Model file for the job. Use its own axes, mm. A direction names the side the tool comes from. Give positions to 0.01 mm unless a question says otherwise; leave off trailing zeros. Loops run counter-clockwise (first coordinate to the right, second up) from the corner with the lowest first, then second, coordinate; pieces in that order, holes last. Notation, with made-up numbers: (31, -39.5) -> (42, -39.5) arc R26 ccw to (42, -21.5) -> close; hole circle Ø6 at (27, 20). An arc over 180 degrees is marked (long way). Use CSV: the item, a comma, the result in double quotes. Start each with the question number.
(1) Cut at A-A on x = -38. Write the cut outline in (y, z), then the cut area to 3 significant figures.
(2) Cut at D-D on z = 58.42. Write the cut outline in (x, y) (3 decimals).
(3) Flat gauge pins, fed straight in: pin 1 (1.4 mm diameter, centred on x = -2, z = 53, fed in from -Y); pin 2 (1 mm diameter, centred on x = -2, y = 1, fed in from +Z); pin 3 (11 mm diameter, centred on y = -20, z = 14, fed in from -X); pin 4 (1 mm diameter, centred on y = -28, z = 19.5, fed in from +X). Where does each tip first touch, or does it go through?
(4) Drill centre lines: probe 1 along X at (y, z) = (-31.5, 11.5); probe 2 along Y at (x, z) = (-26.5, 37.5); probe 3 along Z at (x, y) = (-43, -7.5). Where is each one in solid material? Low to high.
(5) 3-axis set-ups, long thin cutter, end or side, ignore diameter. For faces 1 (the flat face through (-2, -19, 43.18)), 2 (the cylindrical face through (5.924, -16.217, 13.555)), 3 (the cylindrical face through (-51.48, -13.872, 16.349)): which of +Z, -Z, +X, -X, +Y, -Y reach the whole face in a straight line?
(6) Pull direction X, two halves, no side cores. Call faces 4 (the flat face through (-22, 0, 38)), 5 (the conical face through (-43.119, 1.265, 76.464)), 6 (the flat face through (0, -22, 21.3)): pulls with the +X half, pulls with the -X half, needs draft (parallel to the pull), parting line crosses it, or undercut.
(7) Cut at B-B on z = 17.78. Write the cut outline in (x, y), then the cut area to 3 significant figures.
(8) Cut at C-C on y = -12. Write the cut outline in (x, z).
from build123d import *

# Parameters (mm, degrees)
BOSS_EXTRUDE1_DEPTH = 77.47
SKETCH2_W           = 43.18
SKETCH2_H           = 44.45
BOSS_EXTRUDE2_DEPTH = 3.81
SKETCH3_R           = 3.81
SKETCH3_R_2         = 1.27
CUT_EXTRUDE1_DEPTH  = 3.81
SKETCH4_R           = 4.7625
BOSS_EXTRUDE3_DEPTH = 12.7
BOSS_EXTRUDE4_START = 12.7
SKETCH5_R           = 4.7625
BOSS_EXTRUDE4_DEPTH = 12.7
FILLET1_R           = 1.016
SKETCH6_W           = 1.27
SKETCH6_H           = 38.1
CUT_EXTRUDE2_DEPTH  = 1.27
FILLET2_R           = 5.08
CHAMFER1_SIZE       = 2.54


with BuildPart() as part:
    # Sketch1 → Boss-Extrude1 (new body)
    with BuildSketch(Plane.XY):
        Polygon((0, 0), (-41.91, 0), (-41.91, -36.83), (0, -36.83), (0, -40.64), (-41.91, -40.64), (-45.72, -40.64), (-45.72, 0), (-45.72, 3.81), (0, 3.81), align=None)
    extrude(amount=BOSS_EXTRUDE1_DEPTH)

    # Sketch2 → Boss-Extrude2 (add)
    with BuildSketch(Plane(origin=(0, 0, 0), x_dir=(0, 0, -1), z_dir=(1, 0, 0))):
        with Locations((-21.59, -18.415)):
            Rectangle(SKETCH2_W, SKETCH2_H)
    extrude(amount=-BOSS_EXTRUDE2_DEPTH)

    # Sketch3 → Cut-Extrude1 (cut)
    with BuildSketch(Plane.ZY.offset(45.72)):
        with Locations(Location((58.42, -18.415, 0), (0, 0, 270))):
            Circle(SKETCH3_R)
        with Locations(Location((47.244, -7.239, 0), (0, 0, 270))):
            Circle(SKETCH3_R_2)
        with Locations(Location((69.596, -7.239, 0), (0, 0, 270))):
            Circle(SKETCH3_R_2)
        with Locations(Location((69.596, -29.591, 0), (0, 0, 270))):
            Circle(SKETCH3_R_2)
        with Locations(Location((47.244, -29.591, 0), (0, 0, 270))):
            Circle(SKETCH3_R_2)
    extrude(amount=-CUT_EXTRUDE1_DEPTH, mode=Mode.SUBTRACT)

    # Sketch4 → Boss-Extrude3 (add)
    with BuildSketch(Plane.ZY.offset(45.72)):
        with Locations(Location((17.78, -18.415, 0), (0, 0, 90))):
            Circle(SKETCH4_R)
    extrude(amount=BOSS_EXTRUDE3_DEPTH)

    # Sketch5 → Boss-Extrude4 (add)
    with BuildSketch(Plane(origin=(0, 0, 0), x_dir=(0, 0, -1), z_dir=(1, 0, 0)).offset(BOSS_EXTRUDE4_START)):
        with Locations(Location((-17.78, -18.415, 0), (0, 0, 90))):
            Circle(SKETCH5_R)
    extrude(amount=-BOSS_EXTRUDE4_DEPTH)

    # Fillet1
    fillet1_edges = [part.edges().sort_by_distance(p)[0] for p in [
        (-58.42, -23.1775, 17.78),
        (12.7, -23.1775, 17.78),
    ]]
    fillet(fillet1_edges, radius=FILLET1_R)

    # Sketch6 → Cut-Extrude2 (cut)
    with BuildSketch(Plane.XZ):
        with Locations((-1.905, 58.42)):
            Rectangle(SKETCH6_W, SKETCH6_H)
    cut_extrude2 = extrude(amount=-CUT_EXTRUDE2_DEPTH, mode=Mode.SUBTRACT)

    # Mirror1: Cut-Extrude2 across plane
    add(cut_extrude2.mirror(Plane(origin=(0, -18.415, 0), x_dir=(0, 0, 1), z_dir=(0, -1, 0))), mode=Mode.SUBTRACT)

    # Fillet2
    fillet2_edges = [part.edges().sort_by_distance(p)[0] for p in [
        (-45.72, 3.81, 38.735),
        (0, 3.81, 38.735),
        (0, -40.64, 38.735),
        (-45.72, -40.64, 38.735),
    ]]
    fillet(fillet2_edges, radius=FILLET2_R)

    # Chamfer1
    chamfer1_edges = [part.edges().sort_by_distance(p)[0] for p in [
        (-1.969148027, -39.576092628, 77.47),
        (-22.86, -40.64, 77.47),
        (-44.232102448, -39.152102448, 77.47),
        (-45.72, -18.415, 77.47),
        (-1.969148027, 2.746092628, 77.47),
        (-44.232102448, 2.322102448, 77.47),
        (-22.86, 3.81, 77.47),
    ]]
    chamfer(chamfer1_edges, length=CHAMFER1_SIZE)


solid = part.part
Check result:
1,outline,"(-40.64, 0) -> (-36.83, 0) -> (-36.83, 77.47) -> (-38.1, 77.47) -> (-40.64, 74.93) -> close; (0, 0) -> (3.81, 0) -> (3.81, 74.93) -> (1.27, 77.47) -> (0, 77.47) -> close"
1,area,"584 mm²"
2,outline,"(-45.72, -35.56) arc R5.08 ccw to (-40.64, -40.64) -> (-5.08, -40.64) arc R5.08 ccw to (-0.161, -36.83) -> (-1.27, -36.83) -> (-1.27, -38.1) -> (-2.54, -38.1) -> (-2.54, -36.83) -> (-41.91, -36.83) -> (-41.91, -22.225) -> (-45.72, -22.225) -> close; (-45.72, -14.605) -> (-41.91, -14.605) -> (-41.91, 0) -> (-2.54, 0) -> (-2.54, 1.27) -> (-1.27, 1.27) -> (-1.27, 0) -> (-0.161, 0) arc R5.08 ccw to (-5.08, 3.81) -> (-40.64, 3.81) arc R5.08 ccw to (-45.72, -1.27) -> close"
3,pin 1,"y = -40.05"
3,pin 2,"z = 76.33"
3,pin 3,"x = -58.42"
3,pin 4,"x = 0"
4,probe 1,"-45.72 to -41.91, -3.81 to 0"
4,probe 2,"-40.64 to -36.83, 0 to 3.81"
4,probe 3,"0 to 46, 48.49 to 68.35, 70.84 to 77.47"
5,face 1,"+Z, +X"
5,face 2,"+X"
5,face 3,"-X"
6,face 4,"undercut"
6,face 5,"pulls with the -X half"
6,face 6,"pulls with the +X half"
7,outline,"(-58.42, -22.16) arc R1.02 ccw to (-57.4, -23.18) -> (-45.72, -23.18) -> (-45.72, -35.56) arc R5.08 ccw to (-40.64, -40.64) -> (-5.08, -40.64) arc R5.08 ccw to (0, -35.56) -> (0, -23.18) -> (11.68, -23.18) arc R1.02 ccw to (12.7, -22.16) -> (12.7, -14.67) arc R1.02 ccw to (11.68, -13.65) -> (0, -13.65) -> (0, -1.27) arc R5.08 ccw to (-5.08, 3.81) -> (-40.64, 3.81) arc R5.08 ccw to (-45.72, -1.27) -> (-45.72, -13.65) -> (-57.4, -13.65) arc R1.02 ccw to (-58.42, -14.67) -> close; hole (-41.91, -36.83) -> (-3.81, -36.83) -> (-3.81, 0) -> (-41.91, 0) -> close"
7,area,"848 mm²"
8,outline,"(-45.72, 0) -> (-41.91, 0) -> (-41.91, 77.47) -> (-43.18, 77.47) -> (-45.72, 74.93) -> close; (-3.81, 0) -> (0, 0) -> (0, 43.18) -> (-3.81, 43.18) -> close"
